Could you check a few things on this model? Use its own coordinates, in mm. Face numbers are marked on the shaded views. A direction names the side the tool comes from. Coordinates: 2 decimals unless noted, no trailing zeros. Loops run counter-clockwise (first coordinate to the right, second up) from the corner with the lowest first, then second, coordinate; pieces in that order, holes last. Notation, with made-up numbers: (-2.75, 32) - (10.25, 32) arc R21 ccw to (10.25, 66) - close; hole circle Ø5 at (22.25, 5). An arc over 180 degrees is marked (long way). Use CSV: the item, a comma, the result in double quotes.
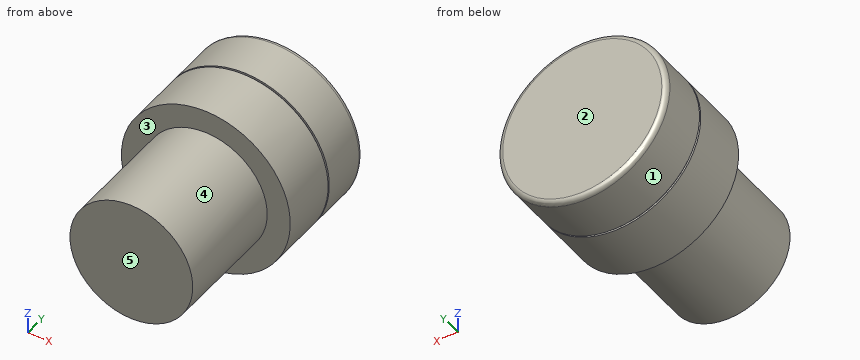
from build123d import *

# Parameters (mm, degrees)
SKETCH1_R      = 8
EXTRUDE1_DEPTH = 15
SKETCH2_R      = 11
EXTRUDE2_DEPTH = 7.62
SKETCH3_R      = 10.75
EXTRUDE3_DEPTH = 0.25
SKETCH4_R      = 11
EXTRUDE4_DEPTH = 6.604
FILLET1_R      = 0.635


with BuildPart() as part:
    # Sketch1 → Extrude1 (new body)
    with BuildSketch(Plane(origin=(0, 0, 0), x_dir=(1, 0, 0), z_dir=(0, 1, 0))):
        with Locations(Location((0, 0, 0), (0, 0, 270))):
            Circle(SKETCH1_R)
    extrude(amount=EXTRUDE1_DEPTH)

    # Sketch2 → Extrude2 (add)
    with BuildSketch(Plane(origin=(0, 15, 0), x_dir=(-1, 0, 0), z_dir=(0, 1, 0))):
        with Locations(Location((0, 0, 0), (0, 0, 270))):
            Circle(SKETCH2_R)
    extrude(amount=EXTRUDE2_DEPTH)

    # Sketch3 → Extrude3 (add)
    with BuildSketch(Plane(origin=(0, 22.62, 0), x_dir=(-1, 0, 0), z_dir=(0, 1, 0))):
        with Locations(Location((0, 0, 0), (0, 0, 90))):
            Circle(SKETCH3_R)
    extrude(amount=EXTRUDE3_DEPTH)

    # Sketch4 → Extrude4 (add)
    with BuildSketch(Plane(origin=(0, 22.87, 0), x_dir=(-1, 0, 0), z_dir=(0, 1, 0))):
        with Locations(Location((0, 0, 0), (0, 0, 270))):
            Circle(SKETCH4_R)
    extrude(amount=EXTRUDE4_DEPTH)

    # Fillet1
    fillet1_edges = [part.edges().sort_by_distance(p)[0] for p in [
        (0, 29.474, 11),
    ]]
    fillet(fillet1_edges, radius=FILLET1_R)


solid = part.part
(1) Please list where these lines run through material, in increasing order: line 1 (Y direction, x = -7, z = 7.25); line 2 (Z direction, x = -2, y = 14.25); line 3 (Z direction, x = -7.5, y = 16.5).
Computed:
line 1,"y = 15 to 29.47"
line 2,"z = -7.75 to 7.75"
line 3,"z = -8.05 to 8.05"
(2) Thinking about a two-plate mould opening in Y: for the marked faces 1, 2 and 3, which applies, +Y half, -Y half, draft (parallel to the pull), parting line (faces both ways), or undercut?
Computed:
face 1,"draft"
face 2,"+Y half"
face 3,"-Y half"
(3) Will these pins go through, and if not, where does the flat tip stop? pin 1 (3 mm diameter, centred on x = 8, y = 19, fed in from -Z); pin 2 (2 mm diameter, centred on y = 23, z = 4.5, fed in from +X); pin 3 (2 mm diameter, centred on x = -8, y = 10, fed in from +Z).
Computed:
pin 1,"stops at z = -8.87"
pin 2,"stops at x = 10.43"
pin 3,"stops at z = 3.87"
(4) Which directions (+Z, -Z, +X, -X, +Y, -Y) give clear straight access to the entire face, cutting with the end or side of a thin tool? Please do the marked faces 4 and 5.
Computed:
face 4,"-Y"
face 5,"+Z, -Z, +X, -X, -Y"
(5) Suppose I cut it at C-C (y = 13). Write out the boundary of the cut face in (x, z), plus the area to 3 significant figures.
Computed:
outline,"circle Ø16 at (0, 0)"
area,"201 mm²"
(6) Suppose I cut it at B-B (z = 0). Write out the boundary of the cut face in (x, y) (3 decimals).
Computed:
outline,"(-11, 15) - (-8, 15) - (-8, 0) - (8, 0) - (8, 15) - (11, 15) - (11, 22.62) - (10.75, 22.62) - (10.75, 22.87) - (11, 22.87) - (11, 28.839) arc R0.635 ccw to (10.365, 29.474) - (-10.365, 29.474) arc R0.635 ccw to (-11, 28.839) - (-11, 22.87) - (-10.75, 22.87) - (-10.75, 22.62) - (-11, 22.62) - close"
(7) Suppose I cut it at A-A (x = 0). Write out the boundary of the cut face in (y, z) (3 decimals), plus the area to 3 significant figures.
Computed:
outline,"(0, -8) - (15, -8) - (15, -11) - (22.62, -11) - (22.62, -10.75) - (22.87, -10.75) - (22.87, -11) - (28.839, -11) arc R0.635 ccw to (29.474, -10.365) - (29.474, 10.365) arc R0.635 ccw to (28.839, 11) - (22.87, 11) - (22.87, 10.75) - (22.62, 10.75) - (22.62, 11) - (15, 11) - (15, 8) - (0, 8) - close"
area,"558 mm²"
